The model under review builds one solid part; all positions refer to its coordinate system, in mm. A direction names the side the tool comes from. Round coordinates to 2 decimals unless told otherwise and drop trailing zeros. Write each loop counter-clockwise with the first axis right and the second up, starting at its lowest first coordinate (ties: lowest second). Pieces come first, ordered by that corner, then holes. Notation, with made-up numbers: (-16.75, -40) - (-2.75, -40) arc R8 cw to (-2.75, -33) - close; hole circle Ø7 at (57.25, 31.5). An arc over 180 degrees is marked (long way). Use one line per item in the form item = value.
from build123d import *

# Parameters (mm, degrees)
PAD012_DEPTH = 110
BOX_W        = 174
BOX_H        = 120
BOX_DEPTH    = 10


with BuildPart() as pad012:
    # Sketch015 → Pad012 (new body)
    with BuildSketch(Plane.XZ.offset(-110)):
        Polygon((10, 12.723166), (10, 8), (5, 8), (5, 2), (175, 2), (175, 8), (170, 8), (170, 13), align=None)
    extrude(amount=PAD012_DEPTH)


with BuildPart() as pcb_holder:
    # Box → Box (new body)
    with BuildSketch(Plane(origin=(3, 0, 0), x_dir=(1, 0, 0), z_dir=(0, 0, 1))):
        with Locations((87, 60)):
            Rectangle(BOX_W, BOX_H)
    extrude(amount=BOX_DEPTH)

    # Cut003: cut Pad012
    add(pad012.part, mode=Mode.SUBTRACT)


with BuildPart() as pcb_holder_1:
    # Cut003 placement: moved
    add(pcb_holder.part.moved(Location((0, -30, 3))))


solid = pcb_holder_1.part
(1) Add section B-B on z = 8.75. Write out the cut boundary in (x, y), then the cut area to 3 significant figures.
Geometry results:
outline = (3, -30) - (5, -30) - (5, 80) - (175, 80) - (175, -30) - (177, -30) - (177, 90) - (3, 90) - close
area = 2,180 mm2
(2) Machinability: for faces 1 (the flat face through (5, 26, 8)), 2 (the flat face through (177, 29, 8)), which of the approach directions +Z, -Z, +X, -X, +Y, -Y give a long, thin tool a straight path to every point of the face, cutting with its end or side? Answer none if there is none.
Geometry results:
face_1 = -Y
face_2 = +Z, -Z, +X, +Y, -Y
(3) To check wall thickness, follow L1, parallel to X at y = 3, z = 9.5; L2, parallel to Y at x = 154, z = 11.5; L3, parallel to Z at x = 78, y = 50. State the ranges of each line that lie inside material, in increasing order.
Geometry results:
L1 = 3 to 5, 175 to 177
L2 = 80 to 90
L3 = 3 to 5
(4) Insertion check: P1, Ø1.5, axis at x = 38.5, z = 8, coming from the -Y side. The pin has a flat end and moves straight along its axis. Give the tip position at first contact, or say it passes through.
Geometry results:
P1 = 80
(5) Add section A-A on y = 54. Write out the cut boundary in (x, z).
Geometry results:
outline = (3, 3) - (177, 3) - (177, 13) - (170, 13) - (170, 11) - (175, 11) - (175, 5) - (5, 5) - (5, 11) - (10, 11) - (10, 13) - (3, 13) - close
(6) The part is to be moulded in two halves that separate along X. For faces 3 (the flat face through (83, 84, 13)), 4 (the flat face through (89, 80, 9)), 5 (the flat face through (3, 29, 8)), 6 (the flat face through (173, 26, 11)), say which applies: +X half, -X half, draft (parallel to the pull), parting line (faces both ways), or undercut.
Geometry results:
face_3 = draft
face_4 = undercut
face_5 = -X half
face_6 = undercut
(7) Add section C-C on x = 116. Write out the cut boundary in (y, z).
Geometry results:
outline = (-30, 3) - (90, 3) - (90, 13) - (80, 13) - (80, 5) - (-30, 5) - close
